Could you check a few things on this model? Use its own coordinates, in mm. A direction names the side the tool comes from. Coordinates: 2 decimals unless noted, no trailing zeros. Loops run counter-clockwise (first coordinate to the right, second up) from the corner with the lowest first, then second, coordinate; pieces in that order, holes last.
from build123d import *

# Parameters (mm, degrees)
F0_W     = 151
F0_H     = 130
F1_DEPTH = 4.8
F2_W     = 99
F2_H     = 29.22
F3_DEPTH = 4.8
F2_R     = 1.55
F4_DEPTH = 4.8
F5_SIZE  = 20
F6_SIZE  = 20
F7_R     = 20
F8_R     = 20


with BuildPart() as f1:
    # F0 (on Front) → F1 (new body)
    with BuildSketch(Plane.XZ):
        Rectangle(F0_W, F0_H)
    extrude(amount=F1_DEPTH)

    # F2 (on face) → F3 (cut)
    with BuildSketch(Plane.XZ.offset(4.8)):
        Rectangle(F2_W, F2_H)
    extrude(amount=-F3_DEPTH, mode=Mode.SUBTRACT)

    # F2 (on face) → F4 (cut)
    with BuildSketch(Plane.XZ.offset(4.8)):
        Rectangle(F2_W, F2_H)
        with Locations((-63.5, -55)):
            Circle(F2_R)
        with Locations((-57.5, -55)):
            Circle(F2_R)
        with Locations((-63.5, -26)):
            Circle(F2_R)
        with Locations((-57.5, -26)):
            Circle(F2_R)
        with Locations((57.5, -26)):
            Circle(F2_R)
        with Locations((63.5, -26)):
            Circle(F2_R)
        with Locations((57.5, -55)):
            Circle(F2_R)
        with Locations((63.5, -55)):
            Circle(F2_R)
        with Locations((-67.5, -16)):
            Circle(F2_R)
        with Locations((67.5, -16)):
            Circle(F2_R)
        with Locations((-58.5, -1)):
            Circle(F2_R)
        with Locations((58.5, -1)):
            Circle(F2_R)
        with Locations((67.5, 43)):
            Circle(F2_R)
        with Locations((-67.5, 43)):
            Circle(F2_R)
        with Locations((-10.5, 45)):
            Circle(F2_R)
        with Locations((10.5, 45)):
            Circle(F2_R)
        with Locations((0.5, 34)):
            Circle(F2_R)
    extrude(amount=-F4_DEPTH, mode=Mode.SUBTRACT)

    # F5
    f5_edges = [f1.edges().sort_by_distance(p)[0] for p in [
        (-75.5, -2.4, 65),
    ]]
    chamfer(f5_edges, length=F5_SIZE)

    # F6
    f6_edges = [f1.edges().sort_by_distance(p)[0] for p in [
        (75.5, -2.4, 65),
    ]]
    chamfer(f6_edges, length=F6_SIZE)

    # F7
    f7_edges = [f1.edges().sort_by_distance(p)[0] for p in [
        (-55.5, -2.4, 65),
    ]]
    fillet(f7_edges, radius=F7_R)

    # F8
    f8_edges = [f1.edges().sort_by_distance(p)[0] for p in [
        (55.5, -2.4, 65),
    ]]
    fillet(f8_edges, radius=F8_R)


solid = f1.part
(1) Imagine slicing it at B-B, the plane x = 36. Write out the boundary of the cut face in (y, z), and give its area (3 significant figures).
Answers:
outline: (-4.8, -65) - (0, -65) - (0, -14.61) - (-4.8, -14.61) - close; (-4.8, 14.61) - (0, 14.61) - (0, 65) - (-4.8, 65) - close
area: 484 mm2
(2) Imagine slicing it at C-C, the plane z = 49. Write out the boundary of the cut face in (x, y).
Answers:
outline: (-71.5, -4.8) - (71.5, -4.8) - (71.5, 0) - (-71.5, 0) - close
(3) Which directions (+Z, -Z, +X, -X, +Y, -Y) give clear straight access to the entire face, cutting with the end or side of a thin tool? Please do faces 1 (the face through (-1, -2, -14.61)), 2 (the face through (-75.5, -2, -11)).
Answers:
face 1: +Y, -Y
face 2: +Z, -Z, -X, +Y, -Y
(4) I need wall thicknesses on probe 1 along Z at (x, y) = (-10.5, -3.7); probe 2 along Z at (x, y) = (26.5, -1.25); probe 3 along Z at (x, y) = (0.5, -2.95). Which ranges of each line are inside material? Lowest first, please.
Answers:
probe 1: z = -65 to -14.61, 14.61 to 43.45, 46.55 to 65
probe 2: z = -65 to -14.61, 14.61 to 65
probe 3: z = -65 to -14.61, 14.61 to 32.45, 35.55 to 65
(5) Imagine slicing it at A-A, the plane y = -3.25. State how many separate pieces and enclosed holes the cut face has, and give its area (3 significant figures).
Answers:
separate pieces: 1
enclosed holes: 18
area: 16,200 mm2
